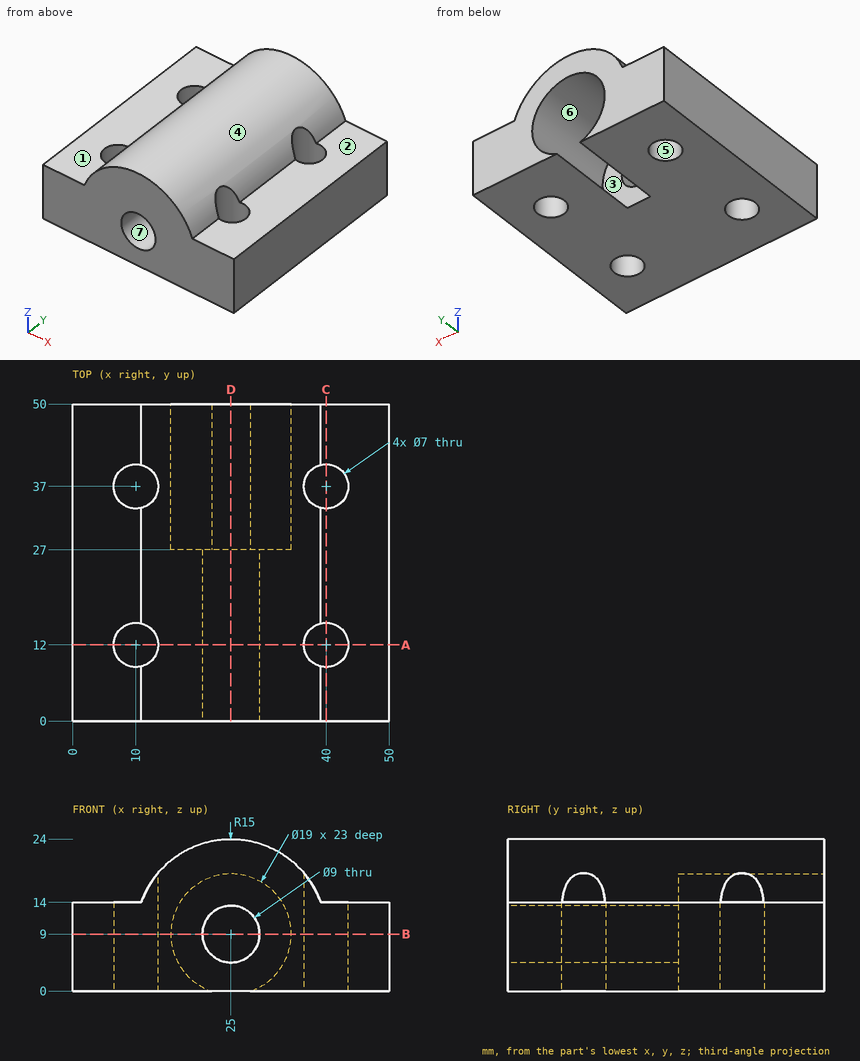
Job drawing, mm, ordinate dimensions from the low corner. One solid piece. A direction names the side the tool comes from. Give positions to 0.01 mm unless a question says otherwise; leave off trailing zeros. Order: outer loops, then holes, each group sorted by start corner. A loop starts at its lowest first (then second) coordinate and runs counter-clockwise, first axis right, second up. Notation, with made-up numbers: M -15,34.25 L 12,34.25 A20 ccw 12,67.25 Z; hole C 15.25,77 d8. An arc over 180 degrees is marked long. Return JSON: item names as keys, results as strings.
Q1. Two-plate mould, pull along Z, no slides. Class the marked faces 4, 5, 6 and 7: pulls with the +Z half, pulls with the -Z half, needs draft (parallel to the pull), parting line crosses it, or undercut.
Answer list:
{"face 4": "pulls with the +Z half", "face 5": "needs draft", "face 6": "undercut", "face 7": "undercut"}
Q2. Flat gauge pins, fed straight in: pin 1 (1.5 mm diameter, centred on y = 9.5, z = 20, fed in from +X); pin 2 (5.5 mm diameter, centred on x = 40, y = 37, fed in from -Z); pin 3 (8 mm diameter, centred on y = 33, z = 17, fed in from -X); pin 4 (9 mm diameter, centred on x = 40, y = 12, fed in from +Z). Where does each tip first touch, or does it go through?
Answer list:
{"pin 1": "stops at x = 35.95", "pin 2": "passes through", "pin 3": "stops at x = 0", "pin 4": "stops at z = 19.71"}
Q3. Wall check: probe 1 along Y at (x, z) = (40, 6); probe 2 along Z at (x, y) = (25, 41.5); probe 3 along Y at (x, z) = (23.5, 16.5). Give the ranges that are in metal, low to high. Write a range as from..to.
Answer list:
{"probe 1": "y = 0..8.5, 15.5..33.5, 40.5..50", "probe 2": "z = 18.5..24", "probe 3": "y = 0..27"}
Q4. Band-saw the part on C-C (x = 40). Give the cut face in (y, z), then the cut area to 3 significant figures.
Answer list:
{"outline": "M 0,0 L 8.5,0 L 8.5,14 L 0,14 Z; M 15.5,0 L 33.5,0 L 33.5,14 L 15.5,14 Z; M 40.5,0 L 50,0 L 50,14 L 40.5,14 Z", "area": "504 mm^2"}
Q5. Band-saw the part on B-B (z = 9). Give the cut face in (x, y), then the cut area to 3 significant figures.
Answer list:
{"outline": "M 0,0 L 20.5,0 L 20.5,27 L 15.5,27 L 15.5,50 L 0,50 Z; M 29.5,0 L 50,0 L 50,50 L 34.5,50 L 34.5,27 L 29.5,27 Z; hole C 10,12 d7; hole C 10,37 d7; hole C 40,12 d7; hole C 40,37 d7", "area": "1,670 mm^2"}
Q6. Band-saw the part on A-A (y = 12). Give the cut face in (x, z), then the cut area to 3 significant figures.
Answer list:
{"outline": "M 0,0 L 6.5,0 L 6.5,14 L 0,14 Z; M 13.5,0 L 36.5,0 L 36.5,18.63 A15 ccw 13.5,18.63 Z; M 43.5,0 L 50,0 L 50,14 L 43.5,14 Z; hole C 25,9 d9", "area": "633 mm^2"}
Q7. 3-axis set-ups, long thin cutter, end or side, ignore diameter. For the marked faces 1, 2 and 3: which of +Z, -Z, +X, -X, +Y, -Y reach the whole face in a straight line?
Answer list:
{"face 1": "+Z, -X, +Y, -Y", "face 2": "+Z, +X, +Y, -Y", "face 3": "+Y"}
Q8. Band-saw the part on D-D (x = 25). Give the cut face in (y, z).
Answer list:
{"outline": "M 0,0 L 27,0 L 27,4.5 L 0,4.5 Z; M 0,13.5 L 27,13.5 L 27,18.5 L 50,18.5 L 50,24 L 0,24 Z"}
